Autodesk Inventor part; units mm, degrees
ref_plane "YZ Plane" through (0, 0, 0) normal (1, 0, 0) x (0, 1, 0)
ref_plane "XZ Plane" through (0, 0, 0) normal (0, 1, 0) x (-1, 0, 0)
ref_plane "XY Plane" through (0, 0, 0) normal (0, 0, 1) x (1, 0, 0)
sketch "Sketch1" plane through (0, 0, 0) normal (0, 0, 1) x (1, 0, 0)
  line L0 (-20.0276, 11.0224) -> (2.5724, 11.0224)
  line L1 (2.5724, 11.0224) -> (2.5724, -8.9776)
  line L2 (2.5724, -8.9776) -> (-20.0276, -8.9776)
  line L3 (-20.0276, -8.9776) -> (-20.0276, 11.0224)
  line L4 (-14.0276, 9.0224) -> (-3.4276, 9.0224)
  line L5 (-3.4276, 9.0224) -> (-3.4276, -6.9776)
  line L6 (-3.4276, -6.9776) -> (-14.0276, -6.9776)
  line L7 (-14.0276, -6.9776) -> (-14.0276, 9.0224)
  point P0 (0, 0)
  point P1 (-20.0276, -6.9776)
  point P2 (-20.0276, 9.0224)
  point P3 (-18.0276, -6.9776)
  point P4 (-18.0276, 9.0224)
  dimension "d0" = 20
  dimension "d1" = 22.6
  dimension "d2" = 2
  dimension "d3" = 6
  dimension "d4" = 6
  dimension "d5" = 2
extrude "Extrusion1" add sketch "Sketch1" along normal blind 2
sketch "Sketch2" plane through (0, 0, 2) normal (0, 0, 1) x (1, 0, 0)
  line L0 (-20.0276, 11.0224) -> (-20.0276, -8.9776)
  line L1 (-20.0276, -8.9776) -> (2.5724, -8.9776)
  line L2 (2.5724, -8.9776) -> (2.5724, 11.0224)
  point P0 (0, 0)
  point P1 (-17.2276, 6.0224)
  point P2 (-17.2276, -5.9776)
  point P3 (-0.2276, 6.0224)
  point P4 (-0.2276, -5.9776)
  dimension "d8" = 2.8
  dimension "d9" = 3
  dimension "d10" = 3
  dimension "d11" = 2.8
  dimension "d12" = 2.8
  dimension "d13" = 2.8
  dimension "d14" = 12
  dimension "d15" = 12
hole "Hole1" at (-17.2276, 6.0224, 2) at (-17.2276, -5.9776, 2) at (-0.2276, 6.0224, 2) at (-0.2276, -5.9776, 2) direction (0, 0, -1) diameter 2 depth 10 tip angle 118
sketch "Sketch3" plane through (0, 0, 2) normal (0, 0, 1) x (1, 0, 0)
  line L0 (-14.0276, -6.9776) -> (-14.0276, 9.0224)
  line L1 (-3.4276, 9.0224) -> (-3.4276, -6.9776)
  line L2 (-14.0276, 9.0224) -> (-3.4276, -6.9776) construction
  line L3 (-14.8612, 8.4701) -> (-4.2612, -7.5299)
  line L4 (-2.5939, -6.4253) -> (-13.1939, 9.5747)
  arc A0 (-13.1939, 9.5747) -> (-14.8612, 8.4701) centre (-14.0276, 9.0224) ccw
  arc A1 (-4.2612, -7.5299) -> (-2.5939, -6.4253) centre (-3.4276, -6.9776) ccw
  line L5 (-3.4276, 9.0224) -> (-14.0276, -6.9776) construction
  line L6 (-4.2612, 9.5747) -> (-14.8612, -6.4253)
  line L7 (-13.1939, -7.5299) -> (-2.5939, 8.4701)
  arc A2 (-2.5939, 8.4701) -> (-4.2612, 9.5747) centre (-3.4276, 9.0224) ccw
  arc A3 (-14.8612, -6.4253) -> (-13.1939, -7.5299) centre (-14.0276, -6.9776) ccw
  point P0 (0, 0)
  point P1 (-8.7276, 1.0224)
  point P2 (-8.7276, 1.0224)
  point P3 (-9.9271, 1.0224)
  point P4 (-8.7276, -0.7882)
  point P5 (-7.528, 1.0224)
  point P6 (-8.7276, 2.833)
  dimension "d23" = 2
  dimension "d24" = 2
extrude "Extrusion2" add sketch "Sketch3" against normal blind 2 contours L6 L3 L7 A3 | L3 A0 L4 L6 | L6 L4 L7 L3 | L7 L4 A1 L3 | L6 A2 L7 L4
fillet "Fillet1" radius 2 4 edges at (-20.0276, 11.0224, 1) (2.5724, 11.0224, 1) (2.5724, -8.9776, 1) (-20.0276, -8.9776, 1)
properties part number "face-2"
Check sheet for the modelled part. Datum: model origin and axes. Units: mm. A direction names the side the tool comes from. Round coordinates to 2 decimals unless told otherwise and drop trailing zeros. Write each loop counter-clockwise with the first axis right and the second up, starting at its lowest first coordinate (ties: lowest second). Pieces come first, ordered by that corner, then holes. Notation, with made-up numbers: (-1.5, -17.5) -> (41.5, -17.5) arc R23 cw to (41.5, 3.5) -> close; hole circle Ø11 at (-0.5, 48). An arc over 180 degrees is marked (long way). One line per question, with ' | ' between items. Start each with the question number.
1. Release check for a two-part mould opening along X. For faces 3 (the face through (-9, 1, 0)), 4 (the face through (-18.22, 6.15, 0.99)), 5 (the face through (-20.028, 1, 1)) record: +X half, -X half, draft (parallel to the pull), parting line (faces both ways), or undercut.
2. Sectioned sample at D-D, the plane z = 1.7. Count the separate pieces of the cut face and the enclosed holes in it, then the cut area to 3 significant figures.
3. Sectioned sample at B-B, the plane x = 0.25. Record the cut outline in (y, z), then the cut area to 3 significant figures.
4. Sectioned sample at A-A, the plane y = 6. Record the cut outline in (x, z).
5. Scan lines: line 1 along X through (y, z) = (5.75, 1.45); line 2 along X through (y, z) = (0.25, 1); line 3 along Y through (x, z) = (-0.5, 1.05). Record each from-to range of solid material in increasing order. Write a range as from..to.
6. Set-up check for faces 1 (the face through (-9, -8.978, 1)), 2 (the face through (-6.65, 5.97, 1.01)): record each of +Z, -Z, +X, -X, +Y, -Y from which the full face is reachable in a straight line by a thin tool's end or side.
7. Sectioned sample at C-C, the plane y = -5.5. Record the cut outline in (x, z), then the cut area to 3 significant figures.
Taken from the geometry:
1) face 3: draft | face 4: undercut | face 5: -X half
2) separate pieces: 1 | enclosed holes: 8 | area: 334 mm^2
3) outline: (-8.98, 0) -> (-6.86, 0) -> (-6.86, 2) -> (-8.98, 2) -> close; (-5.1, 0) -> (5.14, 0) -> (5.14, 2) -> (-5.1, 2) -> close; (6.9, 0) -> (11.02, 0) -> (11.02, 2) -> (6.9, 2) -> close | area: 33.0 mm^2
4) outline: (-20.03, 0) -> (-18.23, 0) -> (-18.23, 2) -> (-20.03, 2) -> close; (-16.23, 0) -> (-14.03, 0) -> (-14.03, 2) -> (-16.23, 2) -> close; (-13.22, 0) -> (-10.83, 0) -> (-10.83, 2) -> (-13.22, 2) -> close; (-6.63, 0) -> (-4.23, 0) -> (-4.23, 2) -> (-6.63, 2) -> close; (-3.43, 0) -> (-1.23, 0) -> (-1.23, 2) -> (-3.43, 2) -> close; (0.77, 0) -> (2.57, 0) -> (2.57, 2) -> (0.77, 2) -> close
5) line 1: x = -20.03..-18.19, -16.27..-14.03, -13.06..-10.66, -6.8..-4.4, -3.43..-1.19, 0.73..2.57 | line 2: x = -20.03..-14.03, -10.44..-7.02, -3.43..2.57 | line 3: y = -8.98..-6.94, -5.02..5.06, 6.98..11.02
6) face 1: +Z, -Z, +X, -X, -Y | face 2: +Z, -Z
7) outline: (-20.03, 0) -> (-18.11, 0) -> (-18.11, 2) -> (-20.03, 2) -> close; (-16.35, 0) -> (-11.85, 0) -> (-11.85, 2) -> (-16.35, 2) -> close; (-5.61, 0) -> (-1.11, 0) -> (-1.11, 2) -> (-5.61, 2) -> close; (0.65, 0) -> (2.57, 0) -> (2.57, 2) -> (0.65, 2) -> close | area: 25.7 mm^2
